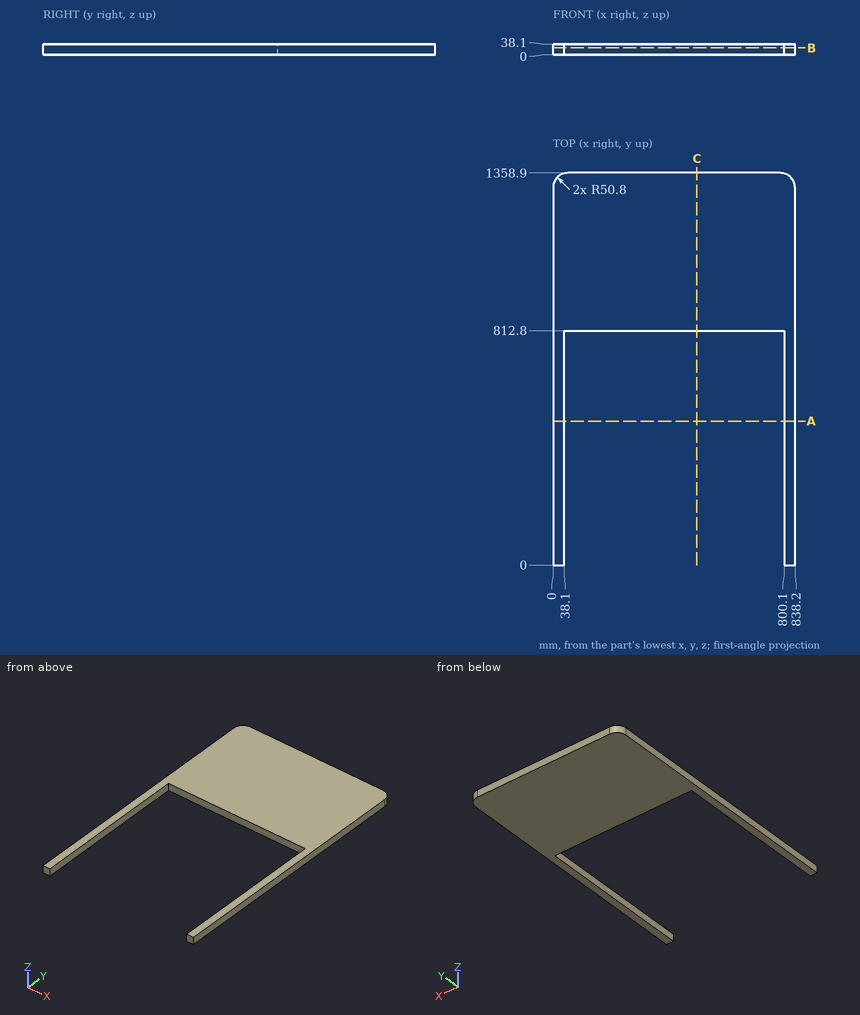
Input: dimensioned drawing with shaded views. Units: mm. Origin: part minimum x, y, z. Give positions to 0.01 mm unless a question says otherwise; leave off trailing zeros. Loops run counter-clockwise (first coordinate to the right, second up) from the corner with the lowest first, then second, coordinate; pieces in that order, holes last. Notation, with made-up numbers: (7.25, 17) -> (62.25, 17) arc R25 ccw to (62.25, 53) -> close; hole circle Ø10 at (-25.5, 63.5). An arc over 180 degrees is marked (long way). Use a Markdown table: item, result. Add a question column.
1) Section query B-B, the plane z = 25. Return the cut outline in (x, y).
2) Section query C-C, the plane x = 498.5. Return the cut outline in (y, z).
3) First-contact query: pin 1 (10 mm diameter, centred on x = 619.5, z = 30.5, fed in from -Y). Flat tip, straight axial feed; report the tip coordinate or a pass-through.
4) Line query: line 1 along X through (y, z) = (352.5, 19); line 2 along Y through (x, z) = (679, 13.5). Output: solid intervals per line, ascending. Write a range as [from, to].
5) Section query A-A, the plane y = 499. Return the cut outline in (x, z).
Numbers:
| question | item | result |
|---|---|---|
| 1 | outline | (0, 0) -> (38.1, 0) -> (38.1, 812.8) -> (800.1, 812.8) -> (800.1, 0) -> (838.2, 0) -> (838.2, 1308.1) arc R50.8 ccw to (787.4, 1358.9) -> (50.8, 1358.9) arc R50.8 ccw to (0, 1308.1) -> close |
| 2 | outline | (812.8, 0) -> (1358.9, 0) -> (1358.9, 38.1) -> (812.8, 38.1) -> close |
| 3 | pin 1 | stops at y = 812.8 |
| 4 | line 1 | x = [0, 38.1], [800.1, 838.2] |
| 4 | line 2 | y = [812.8, 1358.9] |
| 5 | outline | (0, 0) -> (38.1, 0) -> (38.1, 38.1) -> (0, 38.1) -> close; (800.1, 0) -> (838.2, 0) -> (838.2, 38.1) -> (800.1, 38.1) -> close |
